```python
from build123d import *

# Parameters (mm, degrees)
F0_R      = 1.65
F1_DEPTH  = 9.525
F2_R      = 1.65
F3_DEPTH  = 25.4
F4_R      = 3
F4_R_2    = 1.65
F5_DEPTH  = 3.1
F6_R      = 3
F6_R_2    = 1.65
F7_DEPTH  = 3.1
F8_R      = 1.65
F9_DEPTH  = 2.5
F10_R     = 1.65
F11_DEPTH = 2.5
F12_R     = 8.89


with BuildPart() as f1:
    # F0 (on Top) → F1 (new body, symmetric)
    with BuildSketch(Plane.XY):
        with BuildLine():
            Line((22.225, 9.525), (-22.225, 9.525))
            Line((-22.225, 9.525), (-22.225, -9.525))
            Line((-22.225, -9.525), (22.225, -9.525))
            Line((22.225, -9.525), (22.225, -0.635))
            Line((22.225, -0.635), (16.039644, -0.635))
            ThreePointArc((16.039644, -0.635), (0.4445, 0), (16.039644, 0.635))
            Line((16.039644, 0.635), (22.225, 0.635))
            Line((22.225, 0.635), (22.225, 9.525))
        make_face()
        with Locations((-17.78, 0)):
            Circle(F0_R, mode=Mode.SUBTRACT)
    extrude(amount=F1_DEPTH, both=True)

    # F2 (on Front) → F3 (cut, symmetric)
    with BuildSketch(Plane.XZ):
        with BuildLine():
            ThreePointArc((-15.335797, -0.635), (-15.367, 0), (-15.335797, 0.635))
            Line((-15.335797, 0.635), (-22.225, 0.635))
            Line((-22.225, 0.635), (-22.225, -0.635))
            Line((-22.225, -0.635), (-15.335797, -0.635))
        make_face()
        with BuildLine():
            Line((-8.89, 0.635), (-15.335797, 0.635))
            ThreePointArc((-15.335797, 0.635), (-15.367, 0), (-15.335797, -0.635))
            Line((-15.335797, -0.635), (-8.89, -0.635))
            Line((-8.89, -0.635), (-8.89, 0.635))
        make_face()
        with BuildLine():
            ThreePointArc((-15.335797, -0.635), (-8.572117, -6.469195), (-2.413, 0))
            ThreePointArc((-2.413, 0), (-8.572117, 6.469195), (-15.335797, 0.635))
            Line((-15.335797, 0.635), (-8.89, 0.635))
            Line((-8.89, 0.635), (-8.89, -0.635))
            Line((-8.89, -0.635), (-15.335797, -0.635))
        make_face()
        with Locations((18.415, 0)):
            Circle(F2_R)
    extrude(amount=F3_DEPTH, both=True, mode=Mode.SUBTRACT)

    # F4 (on face) → F5 (cut)
    with BuildSketch(Plane.XZ.offset(9.525)):
        with Locations((18.415, 0)):
            Circle(F4_R)
        with Locations((18.415, 0)):
            Circle(F4_R_2, mode=Mode.SUBTRACT)
    extrude(amount=-F5_DEPTH, mode=Mode.SUBTRACT)

    # F6 (on face) → F7 (cut)
    with BuildSketch(Plane.XY.offset(9.525)):
        with Locations((-17.78, 0)):
            Circle(F6_R)
        with Locations((-17.78, 0)):
            Circle(F6_R_2, mode=Mode.SUBTRACT)
    extrude(amount=-F7_DEPTH, mode=Mode.SUBTRACT)

    # F8 (on face) → F9 (cut)
    with BuildSketch(Plane(origin=(0, 9.525, 0), x_dir=(-1, 0, 0), z_dir=(0, 1, 0))):
        Polygon((-16.827287, 2.75), (-20.002713, 2.75), (-21.590426, 0), (-20.002713, -2.75), (-16.827287, -2.75), (-15.239574, 0), align=None)
        with Locations((-18.415, 0)):
            Circle(F8_R, mode=Mode.SUBTRACT)
    extrude(amount=-F9_DEPTH, mode=Mode.SUBTRACT)

    # F10 (on face) → F11 (cut)
    with BuildSketch(Plane(origin=(0, 0, -9.525), x_dir=(1, 0, 0), z_dir=(0, 0, -1))):
        Polygon((-16.192287, 2.75), (-19.367713, 2.75), (-20.955426, 0), (-19.367713, -2.75), (-16.192287, -2.75), (-14.604574, 0), align=None)
        with Locations((-17.78, 0)):
            Circle(F10_R, mode=Mode.SUBTRACT)
    extrude(amount=-F11_DEPTH, mode=Mode.SUBTRACT)

    # F12
    f12_edges = [f1.edges().sort_by_distance(p)[0] for p in [
        (22.225, -5.08, 9.525),
        (22.225, 5.08, 9.525),
        (22.225, -5.08, -9.525),
        (22.225, 5.08, -9.525),
        (-22.225, -9.525, -5.08),
        (-22.225, -9.525, 5.08),
        (-22.225, 9.525, -5.08),
        (-22.225, 9.525, 5.08),
    ]]
    fillet(f12_edges, radius=F12_R)


solid = f1.part
```
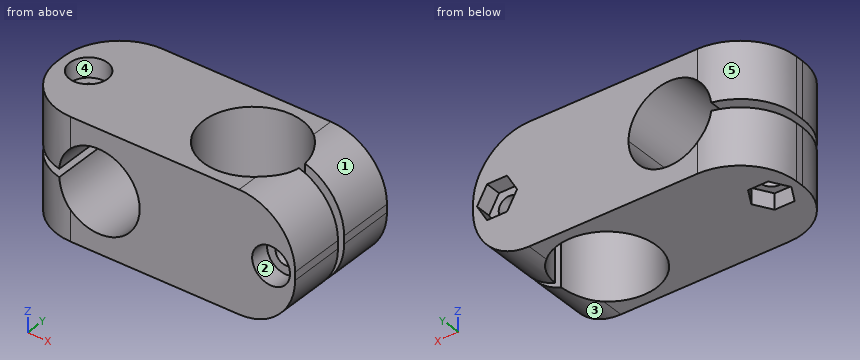
Check sheet for the modelled part. Datum: model origin and axes. Units: mm. Face numbers are marked on the shaded views. A direction names the side the tool comes from. Round coordinates to 2 decimals unless told otherwise and drop trailing zeros. Order: outer loops, then holes, each group sorted by start corner. A loop starts at its lowest first (then second) coordinate and runs counter-clockwise, first axis right, second up. Notation, with made-up numbers: (59, 65) -> (67, 65) arc R14 cw to (67, 83) -> close; hole circle Ø5 at (18.25, 75). An arc over 180 degrees is marked (long way). One line per item, written item: value. Start each with the question number.
Q1. Gauge pin test, flat ends, axial feed: pin 1 Ø4.5 at (x, y) = (-19, 1.5) entering from -Z (3 decimals); pin 2 Ø2 at (x, z) = (18.415, 0) entering from +Y; pin 3 Ø1.8 at (x, y) = (-19, -0.5) entering from +Z (3 decimals); pin 4 Ø5 at (x, y) = (-17.78, 0) entering from -Z (3 decimals). Record the tip position at first contact, or that the pin passes through.
Q2. Cross-section at A-A (x = -8.89). Record the boundary of the cut face in (y, z) (3 decimals).
Q3. Cross-section at C-C (x = -17.78). Record the boundary of the cut face in (y, z) (3 decimals), and give its area (3 significant figures).
Q4. Cross-section at D-D (x = 6.5). Record the boundary of the cut face in (y, z) (3 decimals).
Q5. Mould release check, pull along Z, two halves, no side actions. Record for the marked faces 1, 2 and 3: pulls with the +Z half, pulls with the -Z half, needs draft (parallel to the pull), parting line crosses it, or undercut.
Q6. Thickness scan on line 1 (X direction, y = 0, z = -4.5) (1 decimal); line 2 (X direction, y = -1.75, z = 4.25); line 3 (Z direction, x = -15.5, y = 2) (3 decimals). Record the ranges inside material, lowest first.
Q7. Set-up check for the marked faces 4 and 5: record each of +Z, -Z, +X, -X, +Y, -Y from which the full face is reachable in a straight line by a thin tool's end or side.
Q8. Cross-section at B-B (y = -4). Give the number of separate pieces and of enclosed holes in the cut face, and give its area (3 significant figures).
Completed:
1. pin 1: stops at z = -9.525
1. pin 2: passes through
1. pin 3: stops at z = 6.425
1. pin 4: stops at z = -7.025
2. outline: (-9.525, -9.525) -> (9.525, -9.525) -> (9.525, -6.477) -> (-9.525, -6.477) -> close; (-9.525, 6.477) -> (9.525, 6.477) -> (9.525, 9.525) -> (-9.525, 9.525) -> close
3. outline: (-8.334, -9.525) -> (-2.75, -9.525) -> (-2.75, -7.025) -> (-1.65, -7.025) -> (-1.65, -0.635) -> (-8.334, -0.635) -> close; (-8.334, 0.635) -> (-1.65, 0.635) -> (-1.65, 6.425) -> (-3, 6.425) -> (-3, 9.525) -> (-8.334, 9.525) -> close; (1.65, -7.025) -> (2.75, -7.025) -> (2.75, -9.525) -> (8.334, -9.525) -> (8.334, -0.635) -> (1.65, -0.635) -> close; (1.65, 0.635) -> (8.334, 0.635) -> (8.334, 9.525) -> (3, 9.525) -> (3, 6.425) -> (1.65, 6.425) -> close
3. area: 224 mm²
4. outline: (-9.525, -9.525) -> (-7.611, -9.525) -> (-7.611, 9.525) -> (-9.525, 9.525) -> close; (7.611, -9.525) -> (9.525, -9.525) -> (9.525, 9.525) -> (7.611, 9.525) -> close
5. face 1: pulls with the +Z half
5. face 2: undercut
5. face 3: pulls with the -Z half
6. line 1: x = -22.2 to -19.4, -16.1 to -13.5, -4.2 to 0.4
6. line 2: x = -22.15 to -13.78, -4 to 0.64, 15.87 to 21.46
6. line 3: z = -9.525 to -0.635, 0.635 to 9.525
7. face 4: +Z
7. face 5: +Z, -Z, -X, +Y
8. separate pieces: 2
8. enclosed holes: 1
8. area: 397 mm²
